The model under review builds one solid part; all positions refer to its coordinate system, in mm. Face numbers are marked on the shaded views. A direction names the side the tool comes from. Round coordinates to 2 decimals unless told otherwise and drop trailing zeros. Order: outer loops, then holes, each group sorted by start corner. A loop starts at its lowest first (then second) coordinate and runs counter-clockwise, first axis right, second up. Notation, with made-up numbers: M -9.75,-13.5 L 17.25,-13.5 A28 ccw 17.25,12.5 Z; hole C 33,-32.5 d9. An arc over 180 degrees is marked long. One line per item, written item: value. Start each with the question number.
from build123d import *

# Parameters (mm, degrees)
F1_DEPTH = 30


with BuildPart() as f1:
    # F0 (on Front) → F1 (new body)
    with BuildSketch(Plane.XZ):
        with BuildLine():
            Line((47.193784, 170.781278), (47.193784, 120.781278))
            Line((47.193784, 120.781278), (297.193784, 120.781278))
            Line((297.193784, 120.781278), (297.193784, 370.781278))
            Line((297.193784, 370.781278), (272.193784, 370.781278))
            ThreePointArc((272.193784, 370.781278), (263.65825, 367.245744), (267.193784, 375.781278))
            Line((267.193784, 375.781278), (267.193784, 465.781278))
            ThreePointArc((267.193784, 465.781278), (263.65825, 474.316811), (272.193784, 470.781278))
            Line((272.193784, 470.781278), (297.193784, 470.781278))
            Line((297.193784, 470.781278), (297.193784, 520.781278))
            Line((297.193784, 520.781278), (207.193784, 520.781278))
            Line((207.193784, 520.781278), (207.193784, 475.781278))
            ThreePointArc((207.193784, 475.781278), (210.729318, 467.245744), (202.193784, 470.781278))
            Line((202.193784, 470.781278), (122.193784, 470.781278))
            ThreePointArc((122.193784, 470.781278), (108.051649, 464.923413), (102.193784, 450.781278))
            Line((102.193784, 450.781278), (102.193784, 390.781278))
            ThreePointArc((102.193784, 390.781278), (108.051649, 376.639142), (122.193784, 370.781278))
            Line((122.193784, 370.781278), (202.193784, 370.781278))
            ThreePointArc((202.193784, 370.781278), (210.729318, 374.316811), (207.193784, 365.781278))
            Line((207.193784, 365.781278), (207.193784, 325.781278))
            ThreePointArc((207.193784, 325.781278), (210.729318, 317.245744), (202.193784, 320.781278))
            Line((202.193784, 320.781278), (176.806281, 320.781278))
            ThreePointArc((176.806281, 320.781278), (168.142507, 318.807342), (161.188905, 313.275178))
            Line((161.188905, 313.275178), (47.193784, 170.781278))
        make_face()
        with BuildLine():
            Line((227.193784, 170.781278), (147.980179, 170.781278))
            ThreePointArc((147.980179, 170.781278), (130.022925, 181.975766), (132.167898, 203.027574))
            Line((132.167898, 203.027574), (186.381503, 273.027574))
            ThreePointArc((186.381503, 273.027574), (193.388273, 278.738531), (202.193784, 280.781278))
            Line((202.193784, 280.781278), (227.193784, 280.781278))
            ThreePointArc((227.193784, 280.781278), (241.33592, 274.923413), (247.193784, 260.781278))
            Line((247.193784, 260.781278), (247.193784, 190.781278))
            ThreePointArc((247.193784, 190.781278), (241.33592, 176.639142), (227.193784, 170.781278))
        make_face(mode=Mode.SUBTRACT)
        with BuildLine():
            ThreePointArc((132.167898, 203.027574), (130.022925, 181.975766), (147.980179, 170.781278))
            Line((147.980179, 170.781278), (227.193784, 170.781278))
            ThreePointArc((227.193784, 170.781278), (241.33592, 176.639142), (247.193784, 190.781278))
            Line((247.193784, 190.781278), (247.193784, 260.781278))
            ThreePointArc((247.193784, 260.781278), (241.33592, 274.923413), (227.193784, 280.781278))
            Line((227.193784, 280.781278), (202.193784, 280.781278))
            ThreePointArc((202.193784, 280.781278), (193.388273, 278.738531), (186.381503, 273.027574))
            Line((186.381503, 273.027574), (132.167898, 203.027574))
        make_face()
        with BuildLine():
            ThreePointArc((147.980179, 180.781278), (139.001552, 186.378522), (140.074039, 196.904426))
            Line((140.074039, 196.904426), (194.287644, 266.904426))
            ThreePointArc((194.287644, 266.904426), (197.791028, 269.759904), (202.193784, 270.781278))
            Line((202.193784, 270.781278), (227.193784, 270.781278))
            ThreePointArc((227.193784, 270.781278), (234.264852, 267.852345), (237.193784, 260.781278))
            Line((237.193784, 260.781278), (237.193784, 190.781278))
            ThreePointArc((237.193784, 190.781278), (234.264852, 183.71021), (227.193784, 180.781278))
            Line((227.193784, 180.781278), (147.980179, 180.781278))
        make_face(mode=Mode.SUBTRACT)
    extrude(amount=F1_DEPTH)


solid = f1.part
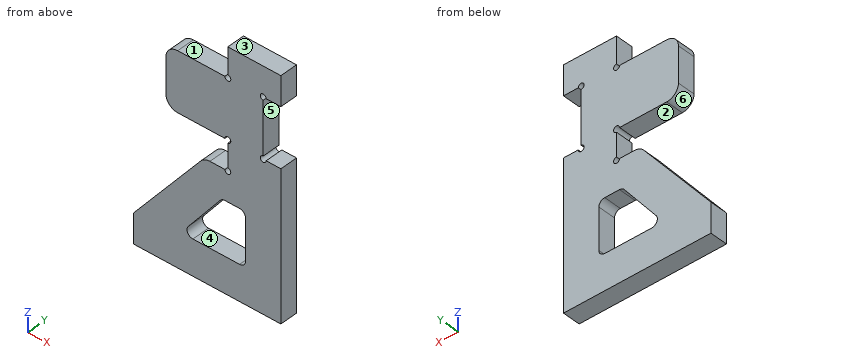
Item 1: Consider section B-B, the plane x = 281.5. Give the boundary of the cut face in (y, z).
Item 2: The part is to be moulded in two halves that separate along X. For the marked faces 4, 5 and 6, say which applies: pulls with the +X half, pulls with the -X half, needs draft (parallel to the pull), parting line crosses it, or undercut.
Item 3: Consider section C-C, the plane z = 186.5. Give the boundary of the cut face in (x, y), then the cut area to 3 significant figures.
Item 4: Wall thickness on L1, parallel to Z at x = 287.5, y = -11.25; L2, parallel to Z at x = 219, y = -13.75; L3, parallel to Z at x = 196, y = -15.75: over which ranges is each line inside the solid? List them lowest first.
Item 5: Consider section D-D, the plane x = 153. Give the boundary of the cut face in (y, z), then the cut area to 3 significant figures.
Item 6: Machinability: for the marked faces 1, 2 and 3, which of the approach directions +Z, -Z, +X, -X, +Y, -Y give a long, thin tool a straight path to every point of the face, cutting with its end or side? Answer none if there is none.
Item 7: Clearance check with flat-ended pins moving along their axes: P1, Ø9, axis at y = -11.5, z = 431.5, coming from the -X side; P2, Ø15, axis at y = -18, z = 403, coming from the +X side; P3, Ø1.5, axis at y = -20, z = 342, coming from the -X side. State where each tip first meets the part, or that it passes through.
Computed:
1. outline: M -30,120.78 L 0,120.78 L 0,370.78 L -30,370.78 Z; M -30,470.78 L 0,470.78 L 0,520.78 L -30,520.78 Z
2. face 4: undercut
2. face 5: pulls with the +X half
2. face 6: pulls with the -X half
3. outline: M 59.77,-30 L 138.94,-30 L 138.94,0 L 59.77,0 Z; M 236.23,-30 L 297.19,-30 L 297.19,0 L 236.23,0 Z
3. area: 4,200 mm^2
4. L1: z = 120.78 to 370.78, 470.78 to 520.78
4. L2: z = 120.78 to 180.78, 270.78 to 520.78
4. L3: z = 120.78 to 180.78, 268.63 to 320.78, 370.78 to 470.78
5. outline: M -30,120.78 L 0,120.78 L 0,180.78 L -30,180.78 Z; M -30,213.59 L 0,213.59 L 0,303.04 L -30,303.04 Z; M -30,370.78 L 0,370.78 L 0,470.78 L -30,470.78 Z
5. area: 7,480 mm^2
6. face 1: +Z, -X, +Y, -Y
6. face 2: -X, +Y, -Y
6. face 3: +Z, +X, -X, +Y, -Y
7. P1: stops at x = 102.19
7. P2: stops at x = 267.19
7. P3: stops at x = 207.19
